Print and shaded views of the part. All mm, measured from the part's lowest x, y and z. A direction names the side the tool comes from. Give positions to 0.01 mm unless a question says otherwise; leave off trailing zeros. Order: outer loops, then holes, each group sorted by start corner. A loop starts at its lowest first (then second) coordinate and runs counter-clockwise, first axis right, second up. Notation, with made-up numbers: (78.5, -24) -> (84.5, -24) arc R19 cw to (84.5, -8) -> close; hole circle Ø2 at (74.25, -33.75). An arc over 180 degrees is marked (long way). One line per question, with ' | ' between items. Start each with the question number.
(1) Pin check, flat tips, straight feed: pin 1 Ø6 at (y, z) = (5, 17) entering from +X; pin 2 Ø1 at (x, y) = (15, 8) entering from -Z; pin 3 Ø11 at (x, z) = (12.5, 15) entering from +Y; pin 4 Ø3 at (x, y) = (26, 21) entering from -Z. Stop position of each tip, or through.
(2) Drill centre lines: L1, parallel to Y at x = 4, z = 2.3; L2, parallel to Z at x = 15, y = 2.8; L3, parallel to Y at x = 28.75, z = 3. Where is each one in solid material? Low to high. Write a range as from..to.
(3) Cut at D-D (z = 10). Give the cut face in (x, y).
(4) Cut at C-C (z = 13). Give the cut face in (x, y), then the cut area to 3 significant figures.
(5) Pull direction X, two halves, no side cores. Call the marked faces 4, 5 and 6: +X half, -X half, draft (parallel to the pull), parting line (faces both ways), or undercut.
(6) Which spindle directions (+Z, -Z, +X, -X, +Y, -Y) get a long thin tool onto all of the face, cutting with end or side? Do the marked faces 1, 2 and 3. Say none if no direction does.
(7) Cut at B-B (x = 15). Give the cut face in (y, z).
(8) Cut at A-A (y = 21). Give the cut face in (x, z).
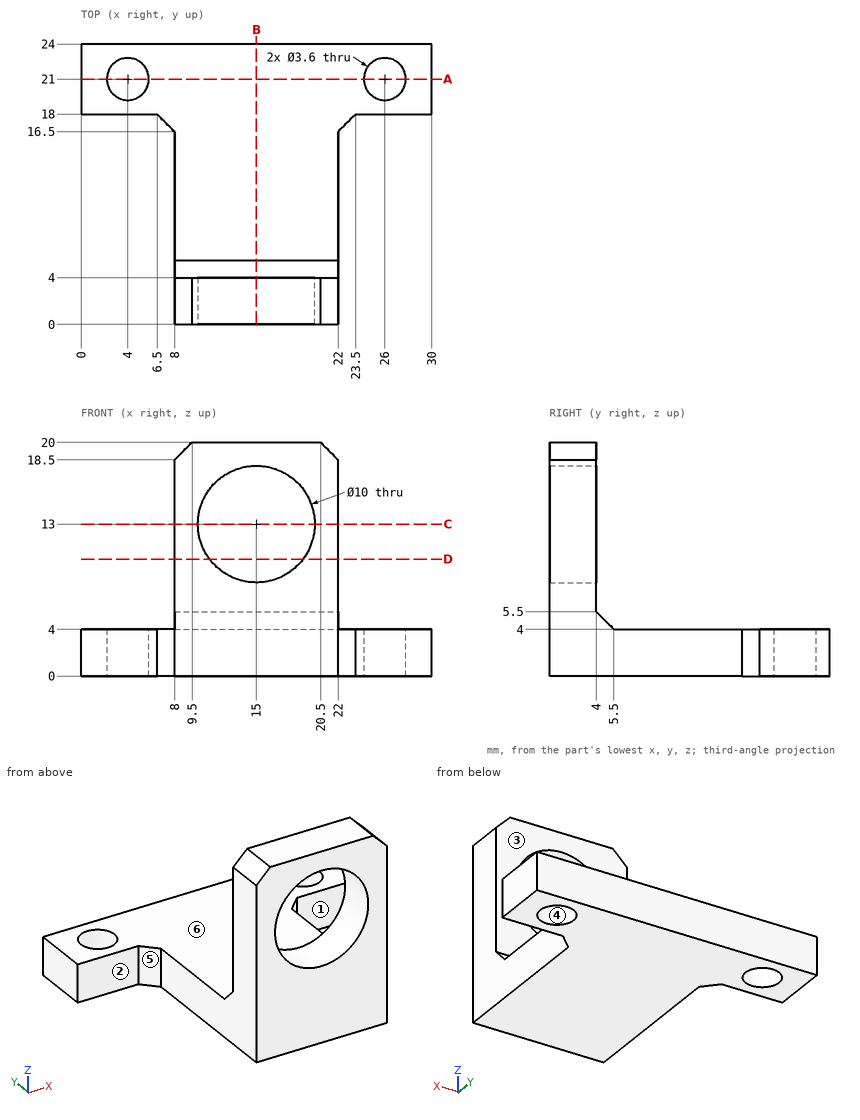
Result set:
1) pin 1: stops at x = 22 | pin 2: stops at z = 0 | pin 3: stops at y = 4 | pin 4: passes through
2) L1: y = 18..19.2, 22.8..24 | L2: z = 0..8, 18..20 | L3: y = 18..24
3) outline: (8, 0) -> (11, 0) -> (11, 4) -> (8, 4) -> close; (19, 0) -> (22, 0) -> (22, 4) -> (19, 4) -> close
4) outline: (8, 0) -> (10, 0) -> (10, 4) -> (8, 4) -> close; (20, 0) -> (22, 0) -> (22, 4) -> (20, 4) -> close | area: 16.0 mm2
5) face 4: undercut | face 5: -X half | face 6: draft
6) face 1: +Z, -Z, +X, -Y | face 2: +Z, -Z, -X, -Y | face 3: +Z, +X, -X, +Y
7) outline: (0, 0) -> (24, 0) -> (24, 4) -> (5.5, 4) -> (4, 5.5) -> (4, 8) -> (0, 8) -> close; (0, 18) -> (4, 18) -> (4, 20) -> (0, 20) -> close
8) outline: (0, 0) -> (2.2, 0) -> (2.2, 4) -> (0, 4) -> close; (5.8, 0) -> (24.2, 0) -> (24.2, 4) -> (5.8, 4) -> close; (27.8, 0) -> (30, 0) -> (30, 4) -> (27.8, 4) -> close
